```python
from build123d import *

# Parameters (mm, degrees)
F0_W     = 142.115966
F0_H     = 120.79817
F1_DEPTH = 127
F2_R     = 14.944743
F3_DEPTH = 127.001
F4_R     = 14.944743
F5_DEPTH = 89.927636


with BuildPart() as f1:
    # F0 (on Front) → F1 (new body)
    with BuildSketch(Plane.XZ):
        with Locations((45.540601, 37.768662)):
            Rectangle(F0_W, F0_H)
    extrude(amount=F1_DEPTH)

    # F2 (on face) → F3 (cut, through all)
    with BuildSketch(Plane.XZ.offset(127)):
        with Locations((68.631113, 58.949754)):
            Circle(F2_R)
    extrude(amount=-F3_DEPTH, mode=Mode.SUBTRACT)

    # F4 (on face) → F5 (join)
    with BuildSketch(Plane.XZ.offset(127)):
        with BuildLine():
            ThreePointArc((-25.517382, 25.873997), (3.077078, 45.820338), (26.239085, 19.762304))
            ThreePointArc((26.239085, 19.762304), (3.077078, -6.295731), (-25.517382, 13.650611))
            Line((-25.517382, 13.650611), (-25.517382, -22.630423))
            Line((-25.517382, -22.630423), (116.598584, -22.630423))
            Line((116.598584, -22.630423), (116.598584, 98.167747))
            Line((116.598584, 98.167747), (-25.517382, 98.167747))
            Line((-25.517382, 98.167747), (-25.517382, 25.873997))
        make_face()
        with Locations((68.631113, 58.949754)):
            Circle(F4_R, mode=Mode.SUBTRACT)
        with BuildLine():
            ThreePointArc((-25.517382, 13.650611), (3.077078, -6.295731), (26.239085, 19.762304))
            ThreePointArc((26.239085, 19.762304), (3.077078, 45.820338), (-25.517382, 25.873997))
            Line((-25.517382, 25.873997), (-25.517382, 13.650611))
        make_face()
    extrude(amount=F5_DEPTH)


solid = f1.part
```
Source: CAD feature listing. Evaluate the final solid. Frame: model axes, mm. Round coordinates to 2 decimals unless told otherwise and drop trailing zeros. Loops run counter-clockwise (first coordinate to the right, second up) from the corner with the lowest first, then second, coordinate; pieces in that order, holes last. Notation, with made-up numbers: M 40.5,9.5 L 78.5,9.5 A18 ccw 78.5,38.5 Z; hole C -23.5,19 d5. An arc over 180 degrees is marked long. Use a Markdown table: item, result. Add a question column.
1. Section query A-A on y = -14. Return the cut outline in (x, z), then the cut area to 3 significant figures.
2. Line query: line 1 (Z direction, x = 64, y = -103); line 2 (Z direction, x = 75, y = -82); line 3 (X direction, y = -206, z = 63.5). Output: solid intervals per line, ascending.
3. Contact query for a flat-ended pin moving along its axis: P1, Ø5, axis at x = 12, z = 50.5, coming from the +Y side. Output: stop coordinate, or through.
Reported:
| question | item | result |
|---|---|---|
| 1 | outline | M -25.52,-22.63 L 116.6,-22.63 L 116.6,98.17 L -25.52,98.17 Z; hole C 68.63,58.95 d29.89 |
| 1 | area | 16,500 mm² |
| 2 | line 1 | z = -22.63 to 44.74, 73.16 to 98.17 |
| 2 | line 2 | z = -22.63 to 45.43, 72.47 to 98.17 |
| 2 | line 3 | x = -25.52 to 54.4, 82.87 to 116.6 |
| 3 | P1 | stops at y = 0 |
